```python
from build123d import *

# Parameters (mm, degrees)
F0_R     = 1.25
F1_DEPTH = 1.25


with BuildPart() as f1:
    # F0 (on Front) → F1 (new body)
    with BuildSketch(Plane.XZ):
        with BuildLine():
            Line((24.5536, 16.676832), (-0.3168, 14.881504))
            ThreePointArc((-0.3168, 14.881504), (-3.338363, 13.359163), (-4.385987, 10.142044))
            Line((-4.385987, 10.142044), (-2.990446, -7.302223))
            ThreePointArc((-2.990446, -7.302223), (-0.008807, -10.062975), (2.98899, -7.319777))
            Line((2.98899, -7.319777), (3.851377, 2.718273))
            ThreePointArc((3.851377, 2.718273), (4.926203, 4.809747), (7.159751, 5.545125))
            Line((7.159751, 5.545125), (24.560498, 4.30852))
            ThreePointArc((24.560498, 4.30852), (25.075008, 4.293377), (25.589, 4.320964))
            Line((25.589, 4.320964), (45.4085, 6.212371))
            ThreePointArc((45.4085, 6.212371), (49.3, 10.492923), (45.4085, 14.773475))
            Line((45.4085, 14.773475), (25.589, 16.664882))
            ThreePointArc((25.589, 16.664882), (25.07155, 16.69251), (24.5536, 16.676832))
        make_face()
        with Locations((0, -7.062988)):
            Circle(F0_R, mode=Mode.SUBTRACT)
        with Locations((0, 10.492923)):
            Circle(F0_R, mode=Mode.SUBTRACT)
        with Locations((25, 10.492923)):
            Circle(F0_R, mode=Mode.SUBTRACT)
        with Locations((39.38, 11.742923)):
            Circle(F0_R, mode=Mode.SUBTRACT)
        with Locations((45, 10.492923)):
            Circle(F0_R, mode=Mode.SUBTRACT)
    extrude(amount=F1_DEPTH)


solid = f1.part
```
Part model, mm, in its own coordinate system. A direction names the side the tool comes from. Round coordinates to 2 decimals unless told otherwise and drop trailing zeros. Loops run counter-clockwise (first coordinate to the right, second up) from the corner with the lowest first, then second, coordinate; pieces in that order, holes last.
Item 1: Cut at D-D, the plane z = -5. Give the cut face in (x, y).
Item 2: Drill centre lines: line 1 (Z direction, x = 0, y = -0.3); line 2 (X direction, y = -0.95, z = 11); line 3 (Z direction, x = -1, y = -0.8). Where is each one in solid material? Low to high.
Item 3: Cut at B-B, the plane y = -0.85. Give the cut face in (x, z).
Item 4: 3-axis set-ups, long thin cutter, end or side, ignore diameter. For faces 4 (the face through (15.738, -0.616, 4.935)), 5 (the face through (16, 0, 9)): which of +Z, -Z, +X, -X, +Y, -Y reach the whole face in a straight line?
Item 5: Cut at C-C, the plane x = 39.38. Give the cut face in (y, z), then the cut area to 3 significant figures.
Item 6: Mould opens along Z. For faces 1 (the face through (44.01, -0.62, 9.73)), 2 (the face through (35.36, -0.616, 5.253)), 3 (the face through (12.29, -0.62, 15.79)) say: +Z half, -Z half, draft (parallel to the pull), parting line (faces both ways), or undercut.
Item 7: Cut at A-A, the plane z = 12.25. Give the cut face in (x, y), then the cut area to 3 significant figures.
A:
1. outline: (-3.17, -1.25) - (3.19, -1.25) - (3.19, 0) - (-3.17, 0) - close
2. line 1: z = -10.06 to -8.31, -5.81 to 9.24, 11.74 to 14.9
2. line 2: x = -4.37 to -1.14, 1.14 to 23.86, 26.14 to 38.37, 40.39 to 43.86, 46.14 to 49.27
2. line 3: z = -9.89 to -7.81, -6.31 to 9.74, 11.24 to 14.78
3. outline: (-4.39, 10.14) - (-2.99, -7.3) arc R3 ccw to (2.99, -7.32) - (3.85, 2.72) arc R3.1 cw to (7.16, 5.55) - (24.56, 4.31) arc R6.2 ccw to (25.59, 4.32) - (45.41, 6.21) arc R4.3 ccw to (45.41, 14.77) - (25.59, 16.66) arc R6.2 ccw to (24.55, 16.68) - (-0.32, 14.88) arc R4.4 ccw to start; hole circle Ø2.5 at (0, -7.06); hole circle Ø2.5 at (0, 10.49); hole circle Ø2.5 at (25, 10.49); hole circle Ø2.5 at (39.38, 11.74); hole circle Ø2.5 at (45, 10.49)
4. face 4: -Z, +Y, -Y
4. face 5: +Z, -Z, +X, -X, +Y
5. outline: (-1.25, 5.64) - (0, 5.64) - (0, 10.49) - (-1.25, 10.49) - close; (-1.25, 12.99) - (0, 12.99) - (0, 15.35) - (-1.25, 15.35) - close
5. area: 9.01 mm2
6. face 1: undercut
6. face 2: -Z half
6. face 3: +Z half
7. outline: (-4.03, -1.25) - (38.24, -1.25) - (38.24, 0) - (-4.03, 0) - close; (40.52, -1.25) - (48.92, -1.25) - (48.92, 0) - (40.52, 0) - close
7. area: 63.3 mm2
